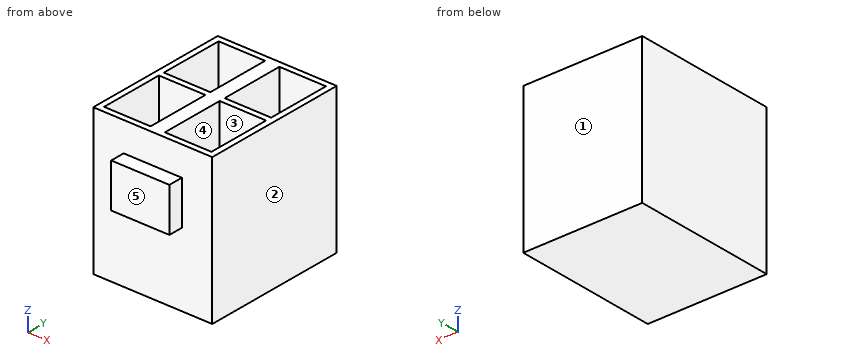
Autodesk Inventor part; units mm, degrees
ref_plane "Work Plane1" through (0, 0, 10) normal (0, 0, 1) x (1, 0, 0)
ref_plane "YZ Plane" through (0, 0, 0) normal (1, 0, 0) x (0, 1, 0)
ref_plane "XZ Plane" through (0, 0, 0) normal (0, 1, 0) x (-1, 0, 0)
sketch "Sketch1" plane through (0, 0, 0) normal (0, 0, 1) x (1, 0, 0)
  line L0 (0, 8) -> (0, -6)
  line L1 (-4.9092, 0) -> (6.5456, 0)
  line L2 (-4.091, 5) -> (4.091, 5)
  line L3 (4.091, 5) -> (4.091, -5)
  line L4 (4.091, -5) -> (-4.091, -5)
  line L5 (-4.091, -5) -> (-4.091, 5)
  dimension "d0" = 8.182
  dimension "d1" = 10
extrude "Extrusion1" add sketch "Sketch1" along normal blind 10
sketch "Sketch5" plane through (-4.091, -5, 0) normal (0, -1, 0) x (1, 0, 0)
  line L0 (8.182, 10) -> (0, 10)
  line L1 (2.091, 8) -> (6.091, 8)
  line L2 (6.091, 8) -> (6.091, 5)
  line L3 (6.091, 5) -> (2.091, 5)
  line L4 (2.091, 5) -> (2.091, 8)
  point P0 (4.091, 8)
  point P1 (4.091, 10)
  dimension "d20" = 4
  dimension "d21" = 3
  dimension "d22" = 2
extrude "Extrusion5" add sketch "Sketch5" along normal blind 1
ref_plane "Work Plane1" through (0, 0, 10) normal (0, 0, 1) x (1, 0, 0)
sketch "Sketch11" plane through (0, 0, 10) normal (0, 0, 1) x (1, 0, 0)
  line L0 (-0.491, -4.6) -> (-3.691, -4.6)
  line L1 (-3.691, -4.6) -> (-3.691, -0.2)
  line L2 (-3.691, -0.2) -> (-0.491, -0.2)
  line L3 (-0.491, -0.2) -> (-0.491, -4.6)
  line L4 (-4.091, -5) -> (-4.091, 5)
  line L5 (4.091, -5) -> (-4.091, -5)
  dimension "d57" = 0.4
  dimension "d58" = 0.4
  dimension "d59" = 3.2
  dimension "d60" = 4.4
extrude "Extrusion11" cut sketch "Sketch11" against normal blind 7
pattern_linear "Rectangular Pattern3" count 2 spacing 4.182 along (1, 0, 0) count 2 spacing 4.8 along (0, 1, 0) of "Extrusion11"
properties part number "Power Supply Header 2"
CAD build for the part. Positions are in the model's coordinates, mm. Face numbers are marked on the shaded views. A direction names the side the tool comes from. Give positions to 0.01 mm unless a question says otherwise; leave off trailing zeros. Write each loop counter-clockwise with the first axis right and the second up, starting at its lowest first coordinate (ties: lowest second). Pieces come first, ordered by that corner, then holes. Notation, with made-up numbers: (83.25, 66) - (114.25, 66) arc R35 cw to (114.25, 101) - close; hole circle Ø10 at (-13, 38.25). An arc over 180 degrees is marked (long way). Put each result on its own line as item: value.
(1) Drop flat-ended pins along their axis: pin 1 Ø2.5 at (x, z) = (-0.5, 4.5) entering from -Y; pin 2 Ø1.6 at (x, y) = (-2.5, 3) entering from +Z. Give the stop position or say it passes through.
Working result:
pin 1: y = -6
pin 2: z = 3
(2) Tool access for the marked faces 4 and 5: list every direction of +Z, -Z, +X, -X, +Y, -Y with a clear straight run to the whole face (end or side of a thin tool).
Working result:
face 4: +Z
face 5: +Z, -Z, +X, -X, -Y
(3) Saw through at C-C (y = -3.5). List the corners of the cut face in (x, z), then the cut area to 3 significant figures.
Working result:
outline: (-4.09, 0) - (4.09, 0) - (4.09, 10) - (3.69, 10) - (3.69, 3) - (0.49, 3) - (0.49, 10) - (-0.49, 10) - (-0.49, 3) - (-3.69, 3) - (-3.69, 10) - (-4.09, 10) - close
area: 37.0 mm^2
(4) Wall check: L1, parallel to X at y = -3.5, z = 8.75; L2, parallel to Y at x = -2.25, z = 7.5; L3, parallel to Y at x = 1.25, z = 6.25. Give the ranges that are in metal, low to high.
Working result:
L1: -4.09 to -3.69, -0.49 to 0.49, 3.69 to 4.09
L2: -5 to -4.6, -0.2 to 0.2, 4.6 to 5
L3: -6 to -4.6, -0.2 to 0.2, 4.6 to 5
(5) Pull direction Y, two halves, no side cores. Call the marked faces 1, 2 and 3: released by +Y, released by -Y, zero draft, split by the parting line, or undercut.
Working result:
face 1: released by +Y
face 2: zero draft
face 3: undercut
(6) Saw through at D-D (z = 7.75). List the corners of the cut face in (x, y).
Working result:
outline: (-4.09, -5) - (-2, -5) - (-2, -6) - (2, -6) - (2, -5) - (4.09, -5) - (4.09, 5) - (-4.09, 5) - close; hole (-3.69, -4.6) - (-0.49, -4.6) - (-0.49, -0.2) - (-3.69, -0.2) - close; hole (-3.69, 0.2) - (-0.49, 0.2) - (-0.49, 4.6) - (-3.69, 4.6) - close; hole (0.49, -4.6) - (3.69, -4.6) - (3.69, -0.2) - (0.49, -0.2) - close; hole (0.49, 0.2) - (3.69, 0.2) - (3.69, 4.6) - (0.49, 4.6) - close
(7) Saw through at B-B (x = -1.75). List the corners of the cut face in (y, z), then the cut area to 3 significant figures.
Working result:
outline: (-6, 5) - (-5, 5) - (-5, 0) - (5, 0) - (5, 10) - (4.6, 10) - (4.6, 3) - (0.2, 3) - (0.2, 10) - (-0.2, 10) - (-0.2, 3) - (-4.6, 3) - (-4.6, 10) - (-5, 10) - (-5, 8) - (-6, 8) - close
area: 41.4 mm^2
(8) Saw through at A-A (z = 3.5). List the corners of the cut face in (x, y).
Working result:
outline: (-4.09, -5) - (4.09, -5) - (4.09, 5) - (-4.09, 5) - close; hole (-3.69, -4.6) - (-0.49, -4.6) - (-0.49, -0.2) - (-3.69, -0.2) - close; hole (-3.69, 0.2) - (-0.49, 0.2) - (-0.49, 4.6) - (-3.69, 4.6) - close; hole (0.49, -4.6) - (3.69, -4.6) - (3.69, -0.2) - (0.49, -0.2) - close; hole (0.49, 0.2) - (3.69, 0.2) - (3.69, 4.6) - (0.49, 4.6) - close
